For this review, take the finished solid that the model builds, in its own axes (mm). A direction names the side the tool comes from. Give positions to 0.01 mm unless a question says otherwise; leave off trailing zeros. Loops run counter-clockwise (first coordinate to the right, second up) from the corner with the lowest first, then second, coordinate; pieces in that order, holes last.
```python
from build123d import *

# Parameters (mm, degrees)
BOSS_EXTRUDE1_DEPTH = 3
FILLET1_R           = 2.5


with BuildPart() as part:
    # Sketch1 → Boss-Extrude1 (new body)
    with BuildSketch(Plane(origin=(0, 0, 0), x_dir=(1, 0, 0), z_dir=(0, 1, 0))):
        with BuildLine():
            Line((-10, 0), (-7.916454192, 0))
            ThreePointArc((-7.916454192, 0), (0, 7.916454192), (7.916454192, 0))
            Line((7.916454192, 0), (10, 0))
            ThreePointArc((10, 0), (0, 10), (-10, 0))
        make_face()
        with BuildLine():
            Line((-7.916454192, -5.916454192), (-7.916454192, 0))
            Line((-7.916454192, 0), (-10, 0))
            ThreePointArc((-10, 0), (-9.464791121, -3.2276507), (-7.916454192, -6.109807936))
            Line((-7.916454192, -6.109807936), (-7.916454192, -5.916454192))
        make_face()
        with BuildLine():
            ThreePointArc((-7.916454192, -6.109807936), (-9.464791121, -3.2276507), (-10, 0))
            Line((-10, 0), (-10, -10))
            Line((-10, -10), (0, -10))
            ThreePointArc((0, -10), (-3.2276507, -9.464791121), (-6.109807936, -7.916454192))
            Line((-6.109807936, -7.916454192), (-7.916454192, -7.916454192))
            Line((-7.916454192, -7.916454192), (-7.916454192, -6.109807936))
        make_face()
        with BuildLine():
            Line((5.916454192, -7.916454192), (0, -7.916454192))
            Line((0, -7.916454192), (-5.916454192, -7.916454192))
            Line((-5.916454192, -7.916454192), (-6.109807936, -7.916454192))
            ThreePointArc((-6.109807936, -7.916454192), (-3.2276507, -9.464791121), (0, -10))
            ThreePointArc((0, -10), (3.2276507, -9.464791121), (6.109807936, -7.916454192))
            Line((6.109807936, -7.916454192), (5.916454192, -7.916454192))
        make_face()
        with BuildLine():
            Line((10, -10), (10, 0))
            ThreePointArc((10, 0), (9.464791121, -3.2276507), (7.916454192, -6.109807936))
            Line((7.916454192, -6.109807936), (7.916454192, -7.916454192))
            Line((7.916454192, -7.916454192), (6.109807936, -7.916454192))
            ThreePointArc((6.109807936, -7.916454192), (3.2276507, -9.464791121), (0, -10))
            Line((0, -10), (10, -10))
        make_face()
        with BuildLine():
            Line((10, 0), (7.916454192, 0))
            Line((7.916454192, 0), (7.916454192, -5.916454192))
            Line((7.916454192, -5.916454192), (7.916454192, -6.109807936))
            ThreePointArc((7.916454192, -6.109807936), (9.464791121, -3.2276507), (10, 0))
        make_face()
        with BuildLine():
            Line((7.916454192, -7.916454192), (7.916454192, -6.109807936))
            ThreePointArc((7.916454192, -6.109807936), (7.071067812, -7.071067812), (6.109807936, -7.916454192))
            Line((6.109807936, -7.916454192), (7.916454192, -7.916454192))
        make_face()
        with BuildLine():
            ThreePointArc((-6.109807936, -7.916454192), (-7.071067812, -7.071067812), (-7.916454192, -6.109807936))
            Line((-7.916454192, -6.109807936), (-7.916454192, -7.916454192))
            Line((-7.916454192, -7.916454192), (-6.109807936, -7.916454192))
        make_face()
    extrude(amount=BOSS_EXTRUDE1_DEPTH)

    # Fillet1
    fillet1_edges = [part.edges().sort_by_distance(p)[0] for p in [
        (-10, 1.5, 10),
        (10, 1.5, 10),
    ]]
    fillet(fillet1_edges, radius=FILLET1_R)


solid = part.part
```
Q1. For pin 1 Ø1.5 at (x, y) = (1.5, 1) entering from -Z; pin 2 Ø1 at (y, z) = (0.5, -8) entering from -X, all flat-tipped, find the tip position at first contact; note any pin that passes through.
Answers:
pin 1: stops at z = -9.97
pin 2: stops at x = -6.61
Q2. For probe 1 along X at (y, z) = (2.75, 5.75); probe 2 along Z at (x, y) = (5.75, 1.8); probe 3 along X at (y, z) = (1.25, -2), list the stretches that pass through material, from the lowest coordinate up.
Answers:
probe 1: x = -10 to -7.92, 7.92 to 10
probe 2: z = -8.18 to -5.44, 7.92 to 10
probe 3: x = -9.8 to -7.66, 7.66 to 9.8
Q3. Consider section B-B on x = 0. Give the boundary of the cut face in (y, z), plus the area to 3 significant figures.
Answers:
outline: (0, -10) - (3, -10) - (3, -7.92) - (0, -7.92) - close; (0, 7.92) - (3, 7.92) - (3, 10) - (0, 10) - close
area: 12.5 mm2
Q4. Consider section A-A on z = 2.75. Give the boundary of the cut face in (x, y).
Answers:
outline: (-10, 0) - (-7.92, 0) - (-7.92, 3) - (-10, 3) - close; (7.92, 0) - (10, 0) - (10, 3) - (7.92, 3) - close
Q5. Mouldability with a two-part tool opening along X and no side actions: class faces 1 (the flat face through (0.7, 0, 8.1)), 2 (the flat face through (-7.916, 1, 3)), 3 (the cylindrical face through (9.287, 1.521, 9.248)), 4 (the flat face through (0, 1, 7.916)) as +X half, -X half, draft (parallel to the pull), parting line (faces both ways), or undercut.
Answers:
face 1: draft
face 2: undercut
face 3: +X half
face 4: undercut
Q6. Consider section D-D on x = -8.25. Give the boundary of the cut face in (y, z).
Answers:
outline: (0, -5.65) - (3, -5.65) - (3, 9.88) - (0, 9.88) - close
Q7. Machinability: for faces 5 (the flat face through (-10, 1, 4)), 6 (the cylindrical face through (-0.174, 1.479, -7.915)), which of the approach directions +Z, -Z, +X, -X, +Y, -Y give a long, thin tool a straight path to every point of the face, cutting with its end or side? Answer none if there is none.
Answers:
face 5: +Z, -Z, -X, +Y, -Y
face 6: +Y, -Y
Q8. Consider section C-C on y = 0.3. Give the boundary of the cut face in (x, z).
Answers:
outline: (-10, 0) arc R10 ccw to (10, 0) - (10, 7.5) arc R2.5 ccw to (7.5, 10) - (-7.5, 10) arc R2.5 ccw to (-10, 7.5) - close; hole (-7.92, 0) arc R7.92 ccw to (7.92, 0) - (7.92, 6.11) arc R10 ccw to (6.11, 7.92) - (-6.11, 7.92) arc R10 ccw to (-7.92, 6.11) - close
